from build123d import *

# Parameters (mm, degrees)
EXTRUDE_START            = -30
EXTRUDE_1_OUTLINE_R      = 15
EXTRUDE_1_DEPTH          = 30
SKETCH_2_W               = 50.000000035
SKETCH_2_H               = 6
EXTRUDE_2_DEPTH          = 30
SKETCH_3_R               = 1.5
CUT_EXTRUDE_1_DEPTH      = 10
SKETCH_4_R               = 3.1
CUT_EXTRUDE_2_DEPTH      = 3
SKETCH_5_R               = 2
CUT_EXTRUDE_3_DEPTH      = 33
CUT_EXTRUDE_4_DEPTH      = 211.848116868
CUT_EXTRUDE_4_DEPTH_BACK = 211.848116868
SKETCH_6_R               = 2


# Read off the part's stored shape, not the designer's step: 填料-伸長1
with BuildPart() as part:
    # 填料-伸長1 outline → 填料-伸長1 (new body)
    with BuildSketch(Plane(origin=(26.04788271, 0, 0), x_dir=(0, 0, -1), z_dir=(1, 0, 0)).offset(EXTRUDE_START)):
        with BuildLine():
            Line((-188, 0.156954032), (-188, -5.64036342))
            ThreePointArc((-188, -5.64036342), (-180, -41.87405136), (-172, -5.64036342))
            Line((-172, -5.64036342), (-172, 0.156954032))
            Line((-172, 0.156954032), (-155, 0.156954032))
            Line((-155, 0.156954032), (-155, 2.156954032))
            Line((-155, 2.156954032), (-205, 2.156954032))
            Line((-205, 2.156954032), (-205, 0.156954032))
            Line((-205, 0.156954032), (-188, 0.156954032))
        make_face()
        with Locations((-180, -22.87405136)):
            Circle(EXTRUDE_1_OUTLINE_R, mode=Mode.SUBTRACT)
    extrude(amount=EXTRUDE_1_DEPTH)

    # 草圖2 → 填料-伸長2 (add)
    with BuildSketch(Plane(origin=(26.04788271, 0, 0), x_dir=(0, 0, -1), z_dir=(1, 0, 0))):
        with Locations((-179.999999983, 5.156954032)):
            Rectangle(SKETCH_2_W, SKETCH_2_H)
    extrude(amount=-EXTRUDE_2_DEPTH)

    # 草圖3 → 除料-伸長1 (cut)
    with BuildSketch(Plane.XZ.offset(-0.156954032)):
        with Locations(Location((19.04788271, 197.5, 0), (0, 0, 270))):
            Circle(SKETCH_3_R)
        with Locations(Location((19.04788271, 162.5, 0), (0, 0, 90))):
            Circle(SKETCH_3_R)
        with Locations(Location((3.04788271, 197.5, 0), (0, 0, 270))):
            Circle(SKETCH_3_R)
        with Locations(Location((3.04788271, 162.5, 0), (0, 0, 90))):
            Circle(SKETCH_3_R)
        with Locations(Location((11.04788271, 197.5, 0), (0, 0, 270))):
            Circle(SKETCH_3_R)
        with Locations(Location((11.04788271, 162.5, 0), (0, 0, 90))):
            Circle(SKETCH_3_R)
    extrude(amount=-CUT_EXTRUDE_1_DEPTH, mode=Mode.SUBTRACT)

    # 草圖4 → 除料-伸長2 (cut)
    with BuildSketch(Plane.XZ.offset(-0.156954032)):
        with Locations(Location((19.04788271, 162.5, 0), (0, 0, 270))):
            Circle(SKETCH_4_R)
        with Locations(Location((3.04788271, 162.5, 0), (0, 0, 270))):
            Circle(SKETCH_4_R)
        with Locations(Location((3.04788271, 197.5, 0), (0, 0, 90))):
            Circle(SKETCH_4_R)
        with Locations(Location((19.04788271, 197.5, 0), (0, 0, 90))):
            Circle(SKETCH_4_R)
        with Locations(Location((11.04788271, 197.5, 0), (0, 0, 270))):
            Circle(SKETCH_4_R)
        with Locations(Location((11.04788271, 162.5, 0), (0, 0, 90))):
            Circle(SKETCH_4_R)
    extrude(amount=-CUT_EXTRUDE_2_DEPTH, mode=Mode.SUBTRACT)

    # 草圖5 → 除料-伸長3 (cut)
    with BuildSketch(Plane(origin=(0, -50, 0), x_dir=(1, 0, 0), z_dir=(0, 1, 0))):
        with Locations(Location((11.04788271, -180, 0), (0, 0, 90))):
            Circle(SKETCH_5_R)
    extrude(amount=CUT_EXTRUDE_3_DEPTH, mode=Mode.SUBTRACT)

    # 草圖6 → 除料-伸長4 (cut, two sides: drawn at the far end of the back side and taken through both)
    with BuildSketch(Plane.XY.offset(-CUT_EXTRUDE_4_DEPTH_BACK)):
        with Locations(Location((11.04788271, -23.75720739, 0), (0, 0, 180))):
            Circle(SKETCH_6_R)
    extrude(amount=CUT_EXTRUDE_4_DEPTH + CUT_EXTRUDE_4_DEPTH_BACK, mode=Mode.SUBTRACT)


solid = part.part
Geometry: final body of the model. Coordinates: model frame, mm. A direction names the side the tool comes from. Round coordinates to 2 decimals unless told otherwise and drop trailing zeros. Order: outer loops, then holes, each group sorted by start corner. A loop starts at its lowest first (then second) coordinate and runs counter-clockwise, first axis right, second up. Notation, with made-up numbers: (25.5, 53) - (71.5, 53) arc R29 cw to (71.5, 86) - close; hole circle Ø10 at (42.25, -24). An arc over 180 degrees is marked (long way). Write each question's results on one line, items separated by ' | '.
Item 1: Mould query, pull axis X, two halves, no side actions, for faces 1 (the cylindrical face through (18.473, 5.622, 196.114)), 2 (the flat face through (26.048, -5, 180)), 3 (the flat face through (8, 0.157, 164)), 4 (the flat face through (12, 3.157, 196)). Classes: pulls with the +X half, pulls with the -X half, needs draft (parallel to the pull), parting line crosses it, or undercut.
Completed:
face 1: undercut | face 2: pulls with the +X half | face 3: needs draft | face 4: undercut
Item 2: Section A-A, the plane z = 162.5. State how many separate pieces and enclosed holes the cut face has, and give its area (3 significant figures).
Completed:
separate pieces: 5 | enclosed holes: 1 | area: 571 mm^2
Item 3: Section C-C, the plane y = -26.5. Return the cut outline in (x, z).
Completed:
outline: (-3.95, 161.35) - (26.05, 161.35) - (26.05, 165.44) - (-3.95, 165.44) - close; (-3.95, 194.56) - (26.05, 194.56) - (26.05, 198.65) - (-3.95, 198.65) - close
Item 4: First-contact query: pin 1 Ø2.5 at (x, z) = (11.05, 162.5) entering from +Y; pin 2 Ø2 at (x, y) = (22, -18) entering from -Z; pin 3 Ø1.9 at (x, z) = (18, 163) entering from -Y; pin 4 Ø3 at (x, y) = (11.05, -23.76) entering from -Z. Flat tips, straight axial feed; report the tip coordinate or a pass-through.
Completed:
pin 1: y = -13.03 | pin 2: z = 161.4 | pin 3: y = -33.04 | pin 4: through
Item 5: Section D-D, the plane x = 15. Return the cut outline in (y, z), and give its area (3 significant figures).
Completed:
outline: (-5.64, 172) - (0.16, 172) - (0.16, 155) - (8.16, 155) - (8.16, 205) - (0.16, 205) - (0.16, 188) - (-5.64, 188) arc R19 ccw (long way) to start; hole circle Ø30 at (-22.87, 180) | area: 901 mm^2
Item 6: Section B-B, the plane z = 180. Return the cut outline in (x, y), and give its area (3 significant figures).
Completed:
outline: (-3.95, -41.87) - (9.05, -41.87) - (9.05, -37.87) - (-3.95, -37.87) - close; (-3.95, -7.87) - (26.05, -7.87) - (26.05, 8.16) - (-3.95, 8.16) - close; (13.05, -41.87) - (26.05, -41.87) - (26.05, -37.87) - (13.05, -37.87) - close | area: 585 mm^2
Item 7: Material intervals for line 1 along X through (y, z) = (1.65, 197.5); line 2 along Y through (x, z) = (11.5, 196); line 3 along X through (y, z) = (4, 162), sorted ascending. Write a range as [from, to].
Completed:
line 1: [-3.95, -0.05], [6.15, 7.95], [14.15, 15.95], [22.15, 26.05] | line 2: [-33.12, -25.71], [-21.81, -12.63], [3.16, 8.16] | line 3: [-3.95, 1.63], [4.46, 9.63], [12.46, 17.63], [20.46, 26.05]
Item 8: Reachability of faces 5 (the cylindrical face through (3.622, 5.622, 163.886)), 6 (the cylindrical face through (2.117, 1.636, 200.457)), 7 (the flat face through (11, 4, 155)), 8 (the cylindrical face through (7.5, -41.86, 180.72)), 9 (the flat face through (14.2, 0.157, 196.6)) from +Z, -Z, +X, -X, +Y, -Y: full face, straight path, thin tool, end or side. Return the list, or none.
Completed:
face 5: +Y | face 6: none | face 7: -Z, +X, -X, +Y, -Y | face 8: +X, -X | face 9: +Z, +X, -X
